Input: part model. Units: mm. Frame: model coordinates. A direction names the side the tool comes from. Coordinates: 2 decimals unless noted, no trailing zeros. Order: outer loops, then holes, each group sorted by start corner. A loop starts at its lowest first (then second) coordinate and runs counter-clockwise, first axis right, second up. Notation, with made-up numbers: M 67,65 L 124,65 A31 ccw 124,92 Z; hole C -25.5,22.5 d8. An arc over 180 degrees is marked long. One line per item, written item: value.
```python
from build123d import *

# Parameters (mm, degrees)
SKETCH1_W                  = 900
SKETCH1_H                  = 2100
BOSS_EXTRUDE1_DEPTH        = 22.5
SKETCH2_W                  = 250
SKETCH2_H                  = 790
SKETCH2_W_2                = 240
SKETCH2_H_2                = 780
CUT_EXTRUDE1_DEPTH         = 15
CHAMFER1_SIZE              = 15
CHAMFER1_OF_MIRROR1_SIZE   = 15
MIRROR2_OUTLINE_W          = 250
MIRROR2_OUTLINE_H          = 790
MIRROR2_OUTLINE_W_2        = 240
MIRROR2_OUTLINE_H_2        = 780
MIRROR2_DEPTH              = 15
MIRROR2_DRAFT              = -45
MIRROR2_2_OUTLINE_W        = 250
MIRROR2_2_OUTLINE_H        = 790
MIRROR2_2_OUTLINE_W_2      = 240
MIRROR2_2_OUTLINE_H_2      = 780
MIRROR2_2_DEPTH            = 15
MIRROR2_2_DRAFT            = -45
CHAMFER2_SIZE              = 15
MIRROR10_COPY_1_SKETCH_W   = 250
MIRROR10_COPY_1_SKETCH_H   = 790
MIRROR10_COPY_1_SKETCH_W_2 = 240
MIRROR10_COPY_1_SKETCH_H_2 = 780
MIRROR10_COPY_1_DEPTH      = 15
MIRROR10_COPY_2_SKETCH_W   = 250
MIRROR10_COPY_2_SKETCH_H   = 790
MIRROR10_COPY_2_SKETCH_W_2 = 240
MIRROR10_COPY_2_SKETCH_H_2 = 780
MIRROR10_COPY_2_DEPTH      = 15
CHAMFER2_OF_MIRROR10_SIZE  = 15
MIRROR11_OUTLINE_W         = 250
MIRROR11_OUTLINE_H         = 790
MIRROR11_OUTLINE_W_2       = 240
MIRROR11_OUTLINE_H_2       = 780
MIRROR11_DEPTH             = 15
MIRROR11_DRAFT             = 45
MIRROR11_2_OUTLINE_W       = 250
MIRROR11_2_OUTLINE_H       = 790
MIRROR11_2_OUTLINE_W_2     = 240
MIRROR11_2_OUTLINE_H_2     = 780
MIRROR11_2_DEPTH           = 15
MIRROR11_2_DRAFT           = 45
SKETCH4_R                  = 27
CUT_EXTRUDE2_DEPTH         = 45


# Read off the part's stored shape, not the designer's step: Mirror2, Mirror11
with BuildPart() as part:
    # Sketch1 → Boss-Extrude1 (new, symmetric)
    with BuildSketch(Plane.XY):
        Rectangle(SKETCH1_W, SKETCH1_H)
    extrude(amount=BOSS_EXTRUDE1_DEPTH, both=True)

    # Sketch2 → Cut-Extrude1 (cut)
    with BuildSketch(Plane.XY.offset(22.5)):
        with Locations((-225, 525)):
            Rectangle(SKETCH2_W, SKETCH2_H)
        with Locations((-225, 525)):
            Rectangle(SKETCH2_W_2, SKETCH2_H_2, mode=Mode.SUBTRACT)
    cut_extrude1 = extrude(amount=-CUT_EXTRUDE1_DEPTH, mode=Mode.SUBTRACT)

    # Chamfer1
    chamfer1_edges = [part.edges().sort_by_distance(p)[0] for p in [
        (-225, 915, 22.5),
        (-105, 525, 22.5),
        (-345, 525, 22.5),
        (-225, 135, 22.5),
        (-225, 920, 22.5),
        (-100, 525, 22.5),
        (-225, 130, 22.5),
        (-350, 525, 22.5),
    ]]
    chamfer(chamfer1_edges, length=CHAMFER1_SIZE - 0.0001)  # a hair under: the kernel refuses the full size

    # Mirror1: Cut-Extrude1 across plane
    add(cut_extrude1.mirror(Plane(origin=(0, 0, 0), x_dir=(0, 0, 1), z_dir=(1, 0, 0))), mode=Mode.SUBTRACT)

    # Chamfer1 of Mirror1
    chamfer1_of_mirror1_edges = [part.edges().sort_by_distance(p)[0] for p in [
        (225, 915, 22.5),
        (105, 525, 22.5),
        (345, 525, 22.5),
        (225, 135, 22.5),
        (225, 920, 22.5),
        (100, 525, 22.5),
        (225, 130, 22.5),
        (350, 525, 22.5),
    ]]
    chamfer(chamfer1_of_mirror1_edges, length=CHAMFER1_OF_MIRROR1_SIZE - 0.0001)  # a hair under: the kernel refuses the full size


with BuildPart() as mirror2_tool:
    # Mirror2 outline → Mirror2 (with draft: the straight prism first)
    with BuildSketch(Plane.XY.offset(7.5)):
        with Locations((-225, -525)):
            Rectangle(MIRROR2_OUTLINE_W, MIRROR2_OUTLINE_H)
        with Locations((-225, -525)):
            Rectangle(MIRROR2_OUTLINE_W_2, MIRROR2_OUTLINE_H_2, mode=Mode.SUBTRACT)
    extrude(amount=MIRROR2_DEPTH)
    # Mirror2: the draft: its side faces are tilted about the plane it starts from
    mirror2_sides = [mirror2_tool.faces().sort_by_distance(p)[0] for p in [
        (-350, -525, 15),
        (-225, -920, 15),
        (-100, -525, 15),
        (-225, -130, 15),
        (-225, -915, 15),
        (-345, -525, 15),
        (-225, -135, 15),
        (-105, -525, 15),
    ]]
    draft(mirror2_sides, Plane.XY.offset(7.5), MIRROR2_DRAFT)


with BuildPart() as part_1:
    add(part.part)

    # Mirror2: cut by mirror2_tool
    add(mirror2_tool.part, mode=Mode.SUBTRACT)


with BuildPart() as mirror2_2_tool:
    # Mirror2 2 outline → Mirror2 2 (with draft: the straight prism first)
    with BuildSketch(Plane.XY.offset(7.5)):
        with Locations((225, -525)):
            Rectangle(MIRROR2_2_OUTLINE_W, MIRROR2_2_OUTLINE_H)
        with Locations((225, -525)):
            Rectangle(MIRROR2_2_OUTLINE_W_2, MIRROR2_2_OUTLINE_H_2, mode=Mode.SUBTRACT)
    extrude(amount=MIRROR2_2_DEPTH)
    # Mirror2 2: the draft: its side faces are tilted about the plane it starts from
    mirror2_2_sides = [mirror2_2_tool.faces().sort_by_distance(p)[0] for p in [
        (350, -525, 15),
        (225, -130, 15),
        (100, -525, 15),
        (225, -920, 15),
        (105, -525, 15),
        (225, -135, 15),
        (345, -525, 15),
        (225, -915, 15),
    ]]
    draft(mirror2_2_sides, Plane.XY.offset(7.5), MIRROR2_2_DRAFT)


with BuildPart() as part_2:
    add(part_1.part)

    # Mirror2 2: cut by mirror2_2_tool
    add(mirror2_2_tool.part, mode=Mode.SUBTRACT)

    # Mirror5: Cut-Extrude1 across plane
    add(cut_extrude1.mirror(Plane.XY), mode=Mode.SUBTRACT)

    # Chamfer2
    chamfer2_edges = [part_2.edges().sort_by_distance(p)[0] for p in [
        (-225, 130, -22.5),
        (-350, 525, -22.5),
        (-100, 525, -22.5),
        (-225, 920, -22.5),
        (-225, 135, -22.5),
        (-345, 525, -22.5),
        (-105, 525, -22.5),
        (-225, 915, -22.5),
    ]]
    chamfer(chamfer2_edges, length=CHAMFER2_SIZE - 0.0001)  # a hair under: the kernel refuses the full size

    # Mirror10 copy 1 sketch → Mirror10 copy 1 (cut)
    with BuildSketch(Plane(origin=(0, 0, -22.5), x_dir=(-1, 0, 0), z_dir=(0, 0, -1))):
        with Locations((-225, 525)):
            Rectangle(MIRROR10_COPY_1_SKETCH_W, MIRROR10_COPY_1_SKETCH_H)
        with Locations((-225, 525)):
            Rectangle(MIRROR10_COPY_1_SKETCH_W_2, MIRROR10_COPY_1_SKETCH_H_2, mode=Mode.SUBTRACT)
    extrude(amount=-MIRROR10_COPY_1_DEPTH, mode=Mode.SUBTRACT)

    # Mirror10 copy 2 sketch → Mirror10 copy 2 (cut)
    with BuildSketch(Plane(origin=(0, 0, 22.5), x_dir=(-1, 0, 0), z_dir=(0, 0, 1))):
        with Locations((-225, -525)):
            Rectangle(MIRROR10_COPY_2_SKETCH_W, MIRROR10_COPY_2_SKETCH_H)
        with Locations((-225, -525)):
            Rectangle(MIRROR10_COPY_2_SKETCH_W_2, MIRROR10_COPY_2_SKETCH_H_2, mode=Mode.SUBTRACT)
    extrude(amount=-MIRROR10_COPY_2_DEPTH, mode=Mode.SUBTRACT)

    # Chamfer2 of Mirror10
    chamfer2_of_mirror10_edges = [part_2.edges().sort_by_distance(p)[0] for p in [
        (225, 130, -22.5),
        (350, 525, -22.5),
        (100, 525, -22.5),
        (225, 920, -22.5),
        (225, 135, -22.5),
        (345, 525, -22.5),
        (105, 525, -22.5),
        (225, 915, -22.5),
    ]]
    chamfer(chamfer2_of_mirror10_edges, length=CHAMFER2_OF_MIRROR10_SIZE - 0.0001)  # a hair under: the kernel refuses the full size


with BuildPart() as mirror11_tool:
    # Mirror11 outline → Mirror11 (with draft: the straight prism first)
    with BuildSketch(Plane.XY.offset(-7.5)):
        with Locations((-225, -525)):
            Rectangle(MIRROR11_OUTLINE_W, MIRROR11_OUTLINE_H)
        with Locations((-225, -525)):
            Rectangle(MIRROR11_OUTLINE_W_2, MIRROR11_OUTLINE_H_2, mode=Mode.SUBTRACT)
    extrude(amount=-MIRROR11_DEPTH)
    # Mirror11: the draft: its side faces are tilted about the plane it starts from
    mirror11_sides = [mirror11_tool.faces().sort_by_distance(p)[0] for p in [
        (-225, -920, -15),
        (-100, -525, -15),
        (-225, -130, -15),
        (-350, -525, -15),
        (-225, -915, -15),
        (-345, -525, -15),
        (-225, -135, -15),
        (-105, -525, -15),
    ]]
    draft(mirror11_sides, Plane.XY.offset(-7.5), MIRROR11_DRAFT)


with BuildPart() as part_3:
    add(part_2.part)

    # Mirror11: cut by mirror11_tool
    add(mirror11_tool.part, mode=Mode.SUBTRACT)


with BuildPart() as mirror11_2_tool:
    # Mirror11 2 outline → Mirror11 2 (with draft: the straight prism first)
    with BuildSketch(Plane.XY.offset(-7.5)):
        with Locations((225, -525)):
            Rectangle(MIRROR11_2_OUTLINE_W, MIRROR11_2_OUTLINE_H)
        with Locations((225, -525)):
            Rectangle(MIRROR11_2_OUTLINE_W_2, MIRROR11_2_OUTLINE_H_2, mode=Mode.SUBTRACT)
    extrude(amount=-MIRROR11_2_DEPTH)
    # Mirror11 2: the draft: its side faces are tilted about the plane it starts from
    mirror11_2_sides = [mirror11_2_tool.faces().sort_by_distance(p)[0] for p in [
        (225, -130, -15),
        (100, -525, -15),
        (225, -920, -15),
        (350, -525, -15),
        (105, -525, -15),
        (225, -135, -15),
        (345, -525, -15),
        (225, -915, -15),
    ]]
    draft(mirror11_2_sides, Plane.XY.offset(-7.5), MIRROR11_2_DRAFT)


with BuildPart() as part_4:
    add(part_3.part)

    # Mirror11 2: cut by mirror11_2_tool
    add(mirror11_2_tool.part, mode=Mode.SUBTRACT)

    # Sketch4 → Cut-Extrude2 (cut)
    with BuildSketch(Plane.XY.offset(22.5)):
        with Locations((350, 0)):
            Circle(SKETCH4_R)
    extrude(amount=-CUT_EXTRUDE2_DEPTH, mode=Mode.SUBTRACT)


solid = part_4.part
```
(1) Draft query along X for faces 1 (the flat face through (450, -15, 0)), 2 (the flat face through (-226, -520, -22.5)), 3 (the flat face through (-450, -15, 0)), 4 (the flat face through (-346, -523, -7.5)). Return one class per face: released by +X, released by -X, zero draft, split by the parting line, or undercut.
Data:
face 1: released by +X
face 2: zero draft
face 3: released by -X
face 4: undercut
(2) Cut plane A-A on y = 0. Output: boundary loops of the cut face in (x, z).
Data:
outline: M -450,-22.5 L 323,-22.5 L 323,22.5 L -450,22.5 Z; M 377,-22.5 L 450,-22.5 L 450,22.5 L 377,22.5 Z
(3) Ray query, line 1 (Y direction, x = 350, z = 6); line 2 (Y direction, x = 97, z = -16); line 3 (X direction, y = 653, z = 19). Return the intervals inside material, ascending. Write a range as from..to.
Data:
line 1: y = -1050..-27, 27..1050
line 2: y = -1050..-928.5, -121.5..121.5, 928.5..1050
line 3: x = -450..-361.5, -333.5..-116.5, -88.5..88.5, 116.5..333.5, 361.5..450
(4) Access query for faces 5 (the cylindrical face through (374.94, -10.34, 0.32)), 6 (the flat face through (-346, 527, 7.5)), 7 (the flat face through (-346, 527, -7.5)). Directions: +Z, -Z, +X, -X, +Y, -Y. A direction counts if a zero-diameter tool reaches every point of the face in a straight line with its end or side. Return the directions, or none.
Data:
face 5: +Z, -Z
face 6: +Z
face 7: -Z
